Geometry: final body of the model. Coordinates: model frame, mm. A direction names the side the tool comes from. Round coordinates to 2 decimals unless told otherwise and drop trailing zeros. Loops run counter-clockwise (first coordinate to the right, second up) from the corner with the lowest first, then second, coordinate; pieces in that order, holes last. Notation, with made-up numbers: (39, -12.5) - (45, -12.5) arc R13 ccw to (45, 7.5) - close; hole circle Ø4 at (10, -18). An arc over 180 degrees is marked (long way). Write item = value, one per line. Start each with the question number.
Item 1: Section B-B (z = -17). Return loops of the section in (x, y).
Item 2: Section C-C (z = -1). Return loops of the section in (x, y), plus the area to 3 significant figures.
Item 3: Draft query along Y for faces 3 (the flat face through (32.5, 10, 6)), 4 (the flat face through (0, 0, 0)), 5 (the flat face through (3, 10, 24)), 6 (the flat face through (0, 20, 0)). Return one class per face: pulls with the +Y half, pulls with the -Y half, needs draft (parallel to the pull), parting line crosses it, or undercut.
Item 4: Access query for faces 1 (the cylindrical face through (42.36, 9.67, -24.493)), 2 (the flat face through (52.5, 10, -17)). Directions: +Z, -Z, +X, -X, +Y, -Y. A direction counts if a zero-diameter tool reaches every point of the face in a straight line with its end or side. Return the directions, or none.
Item 5: Line query: line 1 (X direction, y = 18.5, z = -19); line 2 (Z direction, x = 21, y = 10); line 3 (Z direction, x = 34.5, y = 12). Output: solid intervals per line, ascending. Write a range as from..to.
Item 6: Section D-D (y = 18.75). Return loops of the section in (x, z).
Item 7: First-contact query: pin 1 (1 mm diameter, centred on x = 41.5, z = -19.5, fed in from +Y); pin 2 (12 mm diameter, centred on y = 14.5, z = -2.5, fed in from +X). Flat tips, straight axial feed; report the tip coordinate or a pass-through.
Item 8: Section A-A (y = 10). Return loops of the section in (x, z).
from build123d import *

# Parameters (mm, degrees)
SKETCH2_W           = 65
SKETCH2_H           = 50
BOSS_EXTRUDE1_DEPTH = 20
SKETCH4_W           = 48
SKETCH4_H           = 14
CUT_EXTRUDE1_DEPTH  = 1
SKETCH5_R           = 7.5
BOSS_EXTRUDE2_DEPTH = 20


with BuildPart() as part:
    # Sketch2 → Boss-Extrude1 (new body)
    with BuildSketch(Plane(origin=(0, 0, 0), x_dir=(1, 0, 0), z_dir=(0, 1, 0))):
        Rectangle(SKETCH2_W, SKETCH2_H)
    extrude(amount=BOSS_EXTRUDE1_DEPTH)

    # Sketch4 → Cut-Extrude1 (cut)
    with BuildSketch(Plane.XY.offset(25)):
        with Locations((3.5, 10)):
            Rectangle(SKETCH4_W, SKETCH4_H)
    extrude(amount=-CUT_EXTRUDE1_DEPTH, mode=Mode.SUBTRACT)

    # Sketch5 → Boss-Extrude2 (add)
    with BuildSketch(Plane(origin=(32.5, 0, 0), x_dir=(0, 0, -1), z_dir=(1, 0, 0))):
        with Locations(Location((17, 10, 0), (0, 0, 180))):
            Circle(SKETCH5_R)
    extrude(amount=BOSS_EXTRUDE2_DEPTH)


solid = part.part
Taken from the geometry:
q1.outline = (-32.5, 0) - (32.5, 0) - (32.5, 2.5) - (52.5, 2.5) - (52.5, 17.5) - (32.5, 17.5) - (32.5, 20) - (-32.5, 20) - close
q2.outline = (-32.5, 0) - (32.5, 0) - (32.5, 20) - (-32.5, 20) - close
q2.area = 1,300 mm^2
q3.face_3 = needs draft
q3.face_4 = pulls with the -Y half
q3.face_5 = undercut
q3.face_6 = pulls with the +Y half
q4.face_1 = +X
q4.face_2 = +Z, -Z, +X, +Y, -Y
q5.line_1 = -32.5..32.5
q5.line_2 = -25..24
q5.line_3 = -24.23..-9.77
q6.outline = (-32.5, -25) - (32.5, -25) - (32.5, 25) - (-32.5, 25) - close
q7.pin_1 = 17.23
q7.pin_2 = 32.5
q8.outline = (-32.5, -25) - (32.5, -25) - (32.5, -24.5) - (52.5, -24.5) - (52.5, -9.5) - (32.5, -9.5) - (32.5, 25) - (27.5, 25) - (27.5, 24) - (-20.5, 24) - (-20.5, 25) - (-32.5, 25) - close
